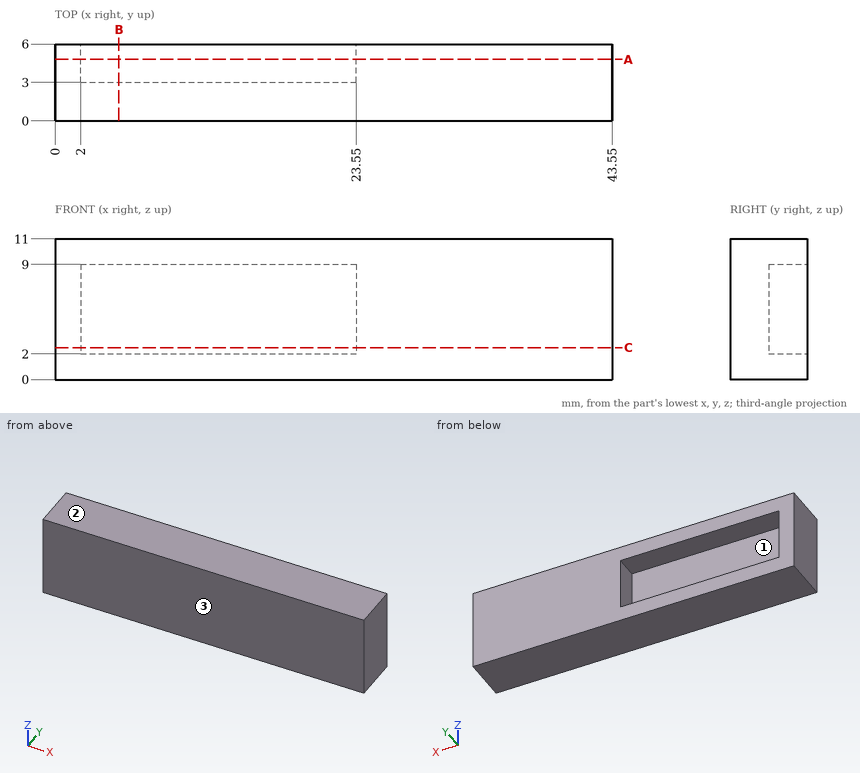
Can you work these out from the drawing? Everything is in mm from the part's minimum corner. Give positions to 0.01 mm unless a question says otherwise; leave off trailing zeros. Order: outer loops, then holes, each group sorted by start corner. A loop starts at its lowest first (then second) coordinate and runs counter-clockwise, first axis right, second up. Notation, with made-up numbers: M 79.5,84 L 104.5,84 A26 ccw 104.5,123 Z; hole C 41,77.5 d6. An arc over 180 degrees is marked long. One line per item, written item: value.
Item 1: If we section it at B-B on x = 5: Write out the boundary of the cut face in (y, z), and give its area (3 significant figures).
Verdict:
outline: M 0,0 L 6,0 L 6,2 L 3,2 L 3,9 L 6,9 L 6,11 L 0,11 Z
area: 45.0 mm2
Item 2: Please list where these lines run through material, in increasing order: line 1 (Z direction, x = 9.5, y = 4.65); line 2 (X direction, y = 3.5, z = 2.75); line 3 (Y direction, x = 5, z = 6.25).
Verdict:
line 1: 0 to 2, 9 to 11
line 2: 0 to 2, 23.55 to 43.55
line 3: 0 to 3
Item 3: If we section it at C-C on z = 2.5: Write out the boundary of the cut face in (x, y).
Verdict:
outline: M 0,0 L 43.55,0 L 43.55,6 L 23.55,6 L 23.55,3 L 2,3 L 2,6 L 0,6 Z
Item 4: For pin 1 (2 mm diameter, centred on x = 16, z = 5.5, fed in from +Y), with a flat end and sliding along its axis, tell me the tip position at first contact or that it passes through.
Verdict:
pin 1: y = 3
Item 5: If we section it at A-A on y = 4.8: Write out the boundary of the cut face in (x, z).
Verdict:
outline: M 0,0 L 43.55,0 L 43.55,11 L 0,11 Z; hole M 2,2 L 23.55,2 L 23.55,9 L 2,9 Z
Item 6: If we mould it in two halves opening along Z, with no side actions, what happens to the marked faces 1, 2 and 3? For each: pulls with the +Z half, pulls with the -Z half, needs draft (parallel to the pull), parting line crosses it, or undercut.
Verdict:
face 1: undercut
face 2: pulls with the +Z half
face 3: needs draft
